Read the model definition and answer for the solid it produces. Units are mm, in the model's axes. Face numbers are marked on the shaded views. Round coordinates to 2 decimals unless told otherwise and drop trailing zeros. Order: outer loops, then holes, each group sorted by start corner. A loop starts at its lowest first (then second) coordinate and runs counter-clockwise, first axis right, second up. Notation, with made-up numbers: (-2, 0) - (41, 0) arc R27 cw to (41, 19) - close; hole circle Ø1 at (22, 35). An arc over 180 degrees is marked (long way). Answer as a JSON object with one key per item and string values. Group by question number.
Q1. The mould has two halves that part along X. Classify the marked faces 1, 2 and 3: pulls with the +X half, pulls with the -X half, needs draft (parallel to the pull), parting line crosses it, or undercut.
Q2. A cutting plane is placed at B-B on y = 1.35. Count the separate pieces of the cut face and the enclosed holes in it, and give its area (3 significant figures).
Q3. A cutting plane is placed at C-C on x = -1.75. Determine the outline of the cut face in (y, z), and give its area (3 significant figures).
Q4. A cutting plane is placed at A-A on z = 0. Determine the outline of the cut face in (x, y).
Q5. Consider line 1 (Z direction, x = 0, y = 2.8); line 2 (Z direction, x = -1, y = 2.1); line 3 (Z direction, x = 0.5, y = 1.4). Determine where each line is inside the solid, lowest interval first.
Q6. A cutting plane is placed at D-D on y = 3.7. Determine the outline of the cut face in (x, z), and give its area (3 significant figures).
Q7. Given pin 1 Ø1 at (y, z) = (0.5, -2) entering from +X; pin 2 Ø4 at (x, z) = (0, 0) entering from -Y; pin 3 Ø2 at (x, z) = (0, -14.625) entering from +Y; pin 4 Ø2 at (x, z) = (0, -5) entering from +Y, each flat-ended and moving along its own axis, determine where each tip first touches the part or whether it passes through.
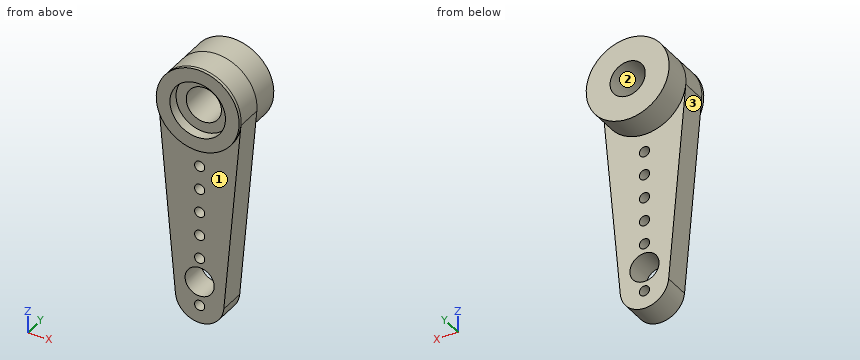
```python
from build123d import *

# Parameters (mm, degrees)
BOSS_EXTRUDE1_DEPTH    = 2.2
SKETCH2_R              = 3.42
BOSS_EXTRUDE2_DEPTH    = 2.33
SKETCH6_R              = 0.42
SKETCH6_R_2            = 0.7
CUT_EXTRUDE5_DEPTH     = 19.547552399
BOSS_EXTRUDE3_START    = 0.27
SKETCH9_R              = 3.42
BOSS_EXTRUDE3_DEPTH    = 0.27
SKETCH10_R             = 2.29
CUT_EXTRUDE12_DEPTH    = 0.85
M2_5_CLEARANCE_HOLE2_D = 2.9
M2_CLEARANCE_HOLE1_D   = 2.4


with BuildPart() as part:
    # Sketch1 → Boss-Extrude1 (new body)
    with BuildSketch(Plane(origin=(0, 0, 0), x_dir=(1, 0, 0), z_dir=(0, 1, 0))):
        with BuildLine():
            Line((-3.406638664, 0.302014925), (-1.992186353, 16.256616915))
            ThreePointArc((-1.992186353, 16.256616915), (0, 18.08), (1.992186353, 16.256616915))
            Line((1.992186353, 16.256616915), (3.406638664, 0.302014925))
            ThreePointArc((3.406638664, 0.302014925), (0, -3.42), (-3.406638664, 0.302014925))
        make_face()
    extrude(amount=BOSS_EXTRUDE1_DEPTH)

    # Sketch2 → Boss-Extrude2 (add)
    with BuildSketch(Plane(origin=(0, 2.2, 0), x_dir=(1, 0, 0), z_dir=(0, 1, 0))):
        with Locations(Location((0, 0, 0), (0, 0, 5.066301357))):
            Circle(SKETCH2_R)
    extrude(amount=BOSS_EXTRUDE2_DEPTH)

    # Sketch6 → Cut-Extrude5 (cut, through all)
    with BuildSketch(Plane(origin=(0, 2.2, 0), x_dir=(1, 0, 0), z_dir=(0, 1, 0))):
        with Locations(Location((0, 4.87, 0), (0, 0, 270))):
            Circle(SKETCH6_R)
        with Locations(Location((0, 6.8125, 0), (0, 0, 270))):
            Circle(SKETCH6_R)
        with Locations(Location((0, 8.755, 0), (0, 0, 270))):
            Circle(SKETCH6_R)
        with Locations(Location((0, 10.6975, 0), (0, 0, 270))):
            Circle(SKETCH6_R)
        with Locations(Location((0, 12.64, 0), (0, 0, 270))):
            Circle(SKETCH6_R)
        with Locations(Location((0, 14.625, 0), (0, 0, 270))):
            Circle(SKETCH6_R_2)
        with Locations(Location((0, 16.61, 0), (0, 0, 270))):
            Circle(SKETCH6_R)
    extrude(amount=-CUT_EXTRUDE5_DEPTH, mode=Mode.SUBTRACT)

    # Sketch9 → Boss-Extrude3 (add)
    with BuildSketch(Plane.XZ.offset(BOSS_EXTRUDE3_START)):
        with Locations(Location((0, 0, 0), (0, 0, 90))):
            Circle(SKETCH9_R)
    extrude(amount=-BOSS_EXTRUDE3_DEPTH)

    # Sketch10 → Cut-Extrude12 (cut)
    with BuildSketch(Plane.XZ.offset(0.27)):
        with Locations(Location((0, 0, 0), (0, 0, 270))):
            Circle(SKETCH10_R)
    extrude(amount=-CUT_EXTRUDE12_DEPTH, mode=Mode.SUBTRACT)

    # M2.5 Clearance Hole2 (through all)
    with Locations(Plane(origin=(0, 0.58, 0), x_dir=(-1, 0, 0), z_dir=(0, -1, 0))):
        with Locations((0, 0)):
            Hole(M2_5_CLEARANCE_HOLE2_D / 2)

    # M2 Clearance Hole1 (through all)
    with Locations(Plane(origin=(0, 0, 0), x_dir=(-1, 0, 0), z_dir=(0, -1, 0))):
        with Locations((0, 14.625)):
            Hole(M2_CLEARANCE_HOLE1_D / 2)


solid = part.part
```
Result set:
{
 "1": {"face 1": "needs draft", "face 2": "undercut", "face 3": "pulls with the -X half"},
 "2": {"separate pieces": "1", "enclosed holes": "8", "area": "97.7 mm²"},
 "3": {"outline": "(-0.27, -2.94) - (0, -2.94) - (0, -17.05) - (2.2, -17.05) - (2.2, -2.94) - (4.53, -2.94) - (4.53, 2.94) - (-0.27, 2.94) - (-0.27, 1.48) - (0.58, 1.48) - (0.58, -1.48) - (-0.27, -1.48) - close", "area": "56.7 mm²"},
 "4": {"outline": "(-3.42, -0.27) - (-2.29, -0.27) - (-2.29, 0.58) - (-1.45, 0.58) - (-1.45, 4.53) - (-3.42, 4.53) - close; (1.45, 0.58) - (2.29, 0.58) - (2.29, -0.27) - (3.42, -0.27) - (3.42, 4.53) - (1.45, 4.53) - close"},
 "5": {"line 1": "z = -3.42 to -1.45, 1.45 to 3.42", "line 2": "z = -17.81 to -15.29, -13.96 to -1.05, 1.05 to 3.27", "line 3": "z = -18.02 to -15.72, -13.53 to -1.36, 1.36 to 3.38"},
 "6": {"outline": "circle Ø6.84 at (0, 0); hole circle Ø2.9 at (0, 0)", "area": "30.1 mm²"},
 "7": {"pin 1": "stops at x = 3.3", "pin 2": "stops at y = 0.58", "pin 3": "passes through", "pin 4": "stops at y = 2.2"}
}
